CAD build for the part. Positions are in the model's coordinates, mm. Face numbers are marked on the shaded views. A direction names the side the tool comes from. Coordinates: 2 decimals unless noted, no trailing zeros. Loops run counter-clockwise (first coordinate to the right, second up) from the corner with the lowest first, then second, coordinate; pieces in that order, holes last. Notation, with made-up numbers: (51, 1.5) -> (70, 1.5) arc R25 cw to (70, 18.5) -> close; hole circle Ø9 at (2.25, -32.75). An arc over 180 degrees is marked (long way). Write each question's results on one line, items separated by ' | '.
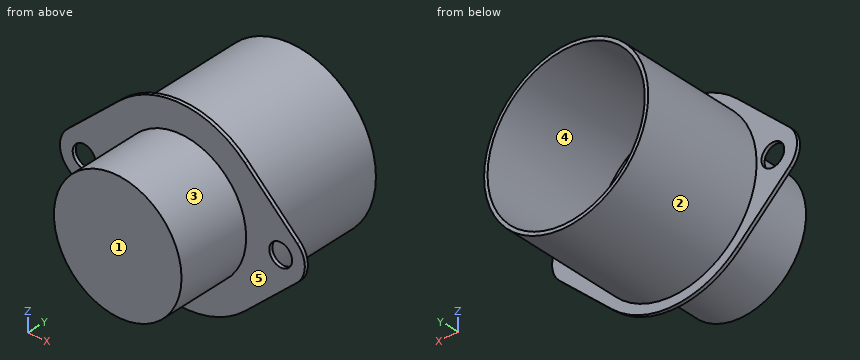
Autodesk Inventor part; units mm, degrees
ref_plane "YZ Plane" through (0, 0, 0) normal (1, 0, 0) x (0, 1, 0)
ref_plane "XZ Plane" through (0, 0, 0) normal (0, 1, 0) x (-1, 0, 0)
ref_plane "XY Plane" through (0, 0, 0) normal (0, 0, 1) x (1, 0, 0)
sketch "Sketch1" plane through (0, 0, 0) normal (0, 1, 0) x (-1, 0, 0)
  line L0 (0, 0) -> (14.25, 0) construction
  circle A0 centre (14.25, 0) radius 1.65
  line L1 (0, 0) -> (17.75, 0) construction
  line L2 (17.75, 0) -> (17.75, -0.5019) construction
  line L3 (9.0658, 9.663) -> (16.6447, 2.5525)
  line L4 (9.0658, -9.663) -> (16.6447, -2.5525)
  arc A1 (16.6447, -2.5525) -> (16.6447, 2.5525) centre (14.25, 0) ccw
  line L5 (0, 0) -> (0, -5) construction
  circle A2 centre (-14.25, 0) radius 1.65
  line L6 (-9.0658, 9.663) -> (-16.6447, 2.5525)
  line L7 (-9.0658, -9.663) -> (-16.6447, -2.5525)
  arc A3 (-16.6447, 2.5525) -> (-16.6447, -2.5525) centre (-14.25, 0) ccw
  arc A4 (9.0658, 9.663) -> (-9.0658, 9.663) centre (0, 0) ccw
  arc A5 (-9.0658, -9.663) -> (9.0658, -9.663) centre (0, 0) ccw
  dimension "d1" = 14.25
  dimension "d2" = 3.3
  dimension "d3" = 17.75
  dimension "d7" = 13.25
  dimension "d8" = 5
extrude "Extrusion1" add sketch "Sketch1" along normal blind 0.5
sketch "Sketch2" plane through (0, 0.5, 0) normal (0, 1, 0) x (1, 0, 0)
  circle A0 centre (0, 0) radius 11.9
  circle A1 centre (0, 0) radius 11.4
  dimension "d11" = 23.8
  dimension "d12" = 22.8
extrude "Extrusion2" add sketch "Sketch2" along normal blind 17.6
sketch "Sketch3" plane through (0, 0, 0) normal (0, -1, 0) x (1, 0, 0)
  circle A0 centre (0, 0) radius 9.25
  dimension "d15" = 18.5
extrude "Extrusion3" add sketch "Sketch3" along normal blind 10.5
properties part number "tube socket 9 pin"
1) Which spindle directions (+Z, -Z, +X, -X, +Y, -Y) get a long thin tool onto all of the face, cutting with end or side? Do the marked faces 1 and 2. Say none if no direction does.
Outcome:
face 1: +Z, -Z, +X, -X, -Y | face 2: +Y
2) Drill centre lines: L1, parallel to Y at x = -10.5, z = -6.75; L2, parallel to Z at x = 0, y = 9.5; L3, parallel to X at y = 2.5, z = -5 (3 decimals). Where is each one in solid material? Low to high. Write a range as from..to.
Outcome:
L1: y = 0..0.5 | L2: z = -11.9..-11.4, 11.4..11.9 | L3: x = -10.799..-10.245, 10.245..10.799
3) Two-plate mould, pull along X, no slides. Class the marked faces 3, 4 and 5: pulls with the +X half, pulls with the -X half, needs draft (parallel to the pull), parting line crosses it, or undercut.
Outcome:
face 3: parting line crosses it | face 4: undercut | face 5: needs draft
4) Slice it at B-B (x = 0). Write the cut outline in (y, z).
Outcome:
outline: (-10.5, -9.25) -> (0, -9.25) -> (0, -13.25) -> (0.5, -13.25) -> (0.5, -11.9) -> (18.1, -11.9) -> (18.1, -11.4) -> (0.5, -11.4) -> (0.5, 11.4) -> (18.1, 11.4) -> (18.1, 11.9) -> (0.5, 11.9) -> (0.5, 13.25) -> (0, 13.25) -> (0, 9.25) -> (-10.5, 9.25) -> close
5) Slice it at D-D (x = 14). Write the cut outline in (y, z), then the cut area to 3 significant figures.
Outcome:
outline: (0, -5.03) -> (0.5, -5.03) -> (0.5, -1.63) -> (0, -1.63) -> close; (0, 1.63) -> (0.5, 1.63) -> (0.5, 5.03) -> (0, 5.03) -> close | area: 3.40 mm^2
6) Slice it at A-A (z = 0). Write the cut outline in (x, y).
Outcome:
outline: (-17.75, 0) -> (-15.9, 0) -> (-15.9, 0.5) -> (-17.75, 0.5) -> close; (-12.6, 0) -> (-9.25, 0) -> (-9.25, -10.5) -> (9.25, -10.5) -> (9.25, 0) -> (12.6, 0) -> (12.6, 0.5) -> (11.9, 0.5) -> (11.9, 18.1) -> (11.4, 18.1) -> (11.4, 0.5) -> (-11.4, 0.5) -> (-11.4, 18.1) -> (-11.9, 18.1) -> (-11.9, 0.5) -> (-12.6, 0.5) -> close; (15.9, 0) -> (17.75, 0) -> (17.75, 0.5) -> (15.9, 0.5) -> close
7) Slice it at C-C (y = 11). Write the cut outline in (x, z), then the cut area to 3 significant figures.
Outcome:
outline: circle Ø23.8 at (0, 0); hole circle Ø22.8 at (0, 0) | area: 36.6 mm^2
8) Pin check, flat tips, straight feed: pin 1 (5 mm diameter, centred on x = -3.5, z = -3, fed in from +Y); pin 2 (1 mm diameter, centred on y = 11, z = -5.5, fed in from -X); pin 3 (1 mm diameter, centred on y = 14, z = -3, fed in from -X). Stop position of each tip, or through.
Outcome:
pin 1: stops at y = 0.5 | pin 2: stops at x = -10.8 | pin 3: stops at x = -11.63
